```python
from build123d import *

# Parameters (mm, degrees)
IZIM1_W                     = 180
IZIM1_H                     = 90
Y_KSEKLIK_EKSTR_ZYON1_DEPTH = 2
IZIM2_W                     = 180
IZIM2_H                     = 1
Y_KSEKLIK_EKSTR_ZYON2_DEPTH = 10
IZIM3_R                     = 2
KES_EKSTR_ZYON1_DEPTH       = 10
IZIM6_W                     = 15
IZIM6_H                     = 25
Y_KSEKLIK_EKSTR_ZYON3_DEPTH = 42
IZIM7_R                     = 3
KES_EKSTR_ZYON2_DEPTH       = 49


with BuildPart() as part:
    # Çizim1 → Yükseklik-Ekstrüzyon1 (new body)
    with BuildSketch(Plane(origin=(0, 0, 0), x_dir=(1, 0, 0), z_dir=(0, 1, 0))):
        Rectangle(IZIM1_W, IZIM1_H)
    extrude(amount=Y_KSEKLIK_EKSTR_ZYON1_DEPTH)

    # Çizim2 → Yükseklik-Ekstrüzyon2 (add)
    with BuildSketch(Plane.XZ):
        with Locations((0, 44.5)):
            Rectangle(IZIM2_W, IZIM2_H)
    y_kseklik_ekstr_zyon2 = extrude(amount=Y_KSEKLIK_EKSTR_ZYON2_DEPTH)

    # Aynalama1: Yükseklik-Ekstrüzyon2 across plane
    add(y_kseklik_ekstr_zyon2.mirror(Plane.XY))

    # Çizim3 → Kes-Ekstrüzyon1 (cut)
    with BuildSketch(Plane.XZ):
        with Locations(Location((-80, 40, 0), (0, 0, 270))):
            Circle(IZIM3_R)
        with Locations(Location((-80, -40, 0), (0, 0, 270))):
            Circle(IZIM3_R)
    kes_ekstr_zyon1 = extrude(amount=-KES_EKSTR_ZYON1_DEPTH, mode=Mode.SUBTRACT)

    # Aynalama2: Kes-Ekstrüzyon1 across plane
    add(kes_ekstr_zyon1.mirror(Plane(origin=(0, 0, 0), x_dir=(0, 0, 1), z_dir=(1, 0, 0))), mode=Mode.SUBTRACT)

    # Çizim6 → Yükseklik-Ekstrüzyon3 (add)
    with BuildSketch(Plane(origin=(0, 2, 0), x_dir=(1, 0, 0), z_dir=(0, 1, 0))):
        with Locations((60.5, 7.5)):
            Rectangle(IZIM6_W, IZIM6_H)
    extrude(amount=Y_KSEKLIK_EKSTR_ZYON3_DEPTH)

    # Çizim7 → Kes-Ekstrüzyon2 (cut)
    with BuildSketch(Plane.ZY.offset(-53)):
        with Locations((-7.5, 39)):
            Circle(IZIM7_R)
    extrude(amount=-KES_EKSTR_ZYON2_DEPTH, mode=Mode.SUBTRACT)


solid = part.part
```
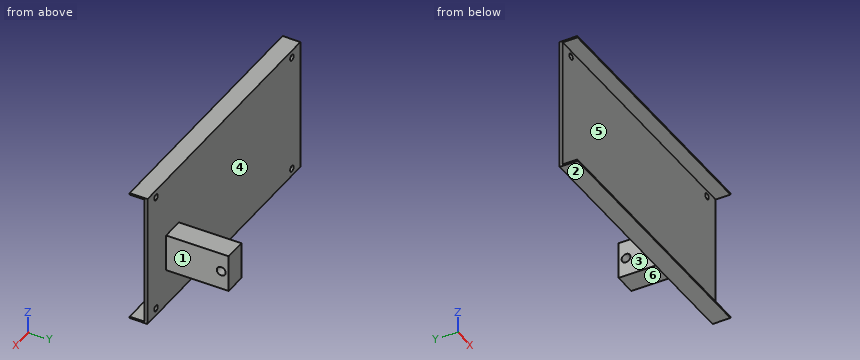
Read the model definition and answer for the solid it produces. Units are mm, in the model's axes. Face numbers are marked on the shaded views. A direction names the side the tool comes from. Coordinates: 2 decimals unless noted, no trailing zeros. Order: outer loops, then holes, each group sorted by start corner. A loop starts at its lowest first (then second) coordinate and runs counter-clockwise, first axis right, second up. Notation, with made-up numbers: (-6.5, 7) - (29.5, 7) arc R13 cw to (29.5, 20) - close; hole circle Ø8 at (-10, 83). An arc over 180 degrees is marked (long way). Answer as a JSON object with one key per item and string values. Group by question number.
Item 1: Flat-ended cylindrical pins translate along their axes: P1, Ø8, axis at x = -35.5, z = -27.5, coming from the +Y side; P2, Ø1.5, axis at x = -42.5, z = 2, coming from the -Y side; P3, Ø12, axis at x = 61.5, y = 21.5, coming from the -Z side; P4, Ø5.5, axis at y = 39, z = -7.5, coming from the -X side. Find the tip coordinate at first contact, or state that the pin passes through.
Item 2: A tool of negligible diameter and unlimited length cuts with its end or side. For the marked faces 1, 2 and 3, from which of +Z, -Z, +X, -X, +Y, -Y can it reach the whole face along a straight path? Write none if from no direction.
Item 3: Section D-D (x = -10) is taken. Give the vertices of the cut face in (y, z), plus the area to 3 significant figures.
Item 4: Section C-C (z = -7.5) is taken. Give the vertices of the cut face in (x, y), plus the area to 3 significant figures.
Item 5: Consider probe 1 along Z at (x, y) = (80, 1.05); probe 2 along X at (y, z) = (0.95, 40); probe 3 along Z at (x, y) = (65, -0.5). Determine where each line is inside the solid, lowest interval first. Write a range as from..to.
Item 6: Section A-A (x = -80) is taken. Give the vertices of the cut face in (y, z).
Item 7: Section B-B (y = 39) is taken. Give the vertices of the cut face in (x, z), plus the area to 3 significant figures.
Item 8: The mould has two halves that part along Z. Classify the marked faces 4, 5 and 6: +Z half, -Z half, draft (parallel to the pull), parting line (faces both ways), or undercut.
Results are:
{
 "1": {"P1": "stops at y = 2", "P2": "stops at y = 0", "P3": "stops at z = -20", "P4": "passes through"},
 "2": {"face 1": "+Z, -Z, +X, +Y", "face 2": "-Z, +X, -X, +Y, -Y", "face 3": "+Z, -Z, -X, +Y"},
 "3": {"outline": "(-10, -45) - (2, -45) - (2, 45) - (-10, 45) - (-10, 44) - (0, 44) - (0, -44) - (-10, -44) - close", "area": "200 mm^2"},
 "4": {"outline": "(-90, 0) - (90, 0) - (90, 2) - (68, 2) - (68, 36) - (53, 36) - (53, 2) - (-90, 2) - close; (53, 42) - (68, 42) - (68, 44) - (53, 44) - close", "area": "900 mm^2"},
 "5": {"probe 1": "z = -45..-42, -38..38, 42..45", "probe 2": "x = -90..-82, -78..78, 82..90", "probe 3": "z = -45..-44, 44..45"},
 "6": {"outline": "(-10, -45) - (2, -45) - (2, -42) - (0, -42) - (0, -44) - (-10, -44) - close; (-10, 44) - (0, 44) - (0, 42) - (2, 42) - (2, 45) - (-10, 45) - close; (0, -38) - (2, -38) - (2, 38) - (0, 38) - close"},
 "7": {"outline": "(53, -20) - (68, -20) - (68, -10.5) - (53, -10.5) - close; (53, -4.5) - (68, -4.5) - (68, 5) - (53, 5) - close", "area": "285 mm^2"},
 "8": {"face 4": "draft", "face 5": "undercut", "face 6": "-Z half"}
}
